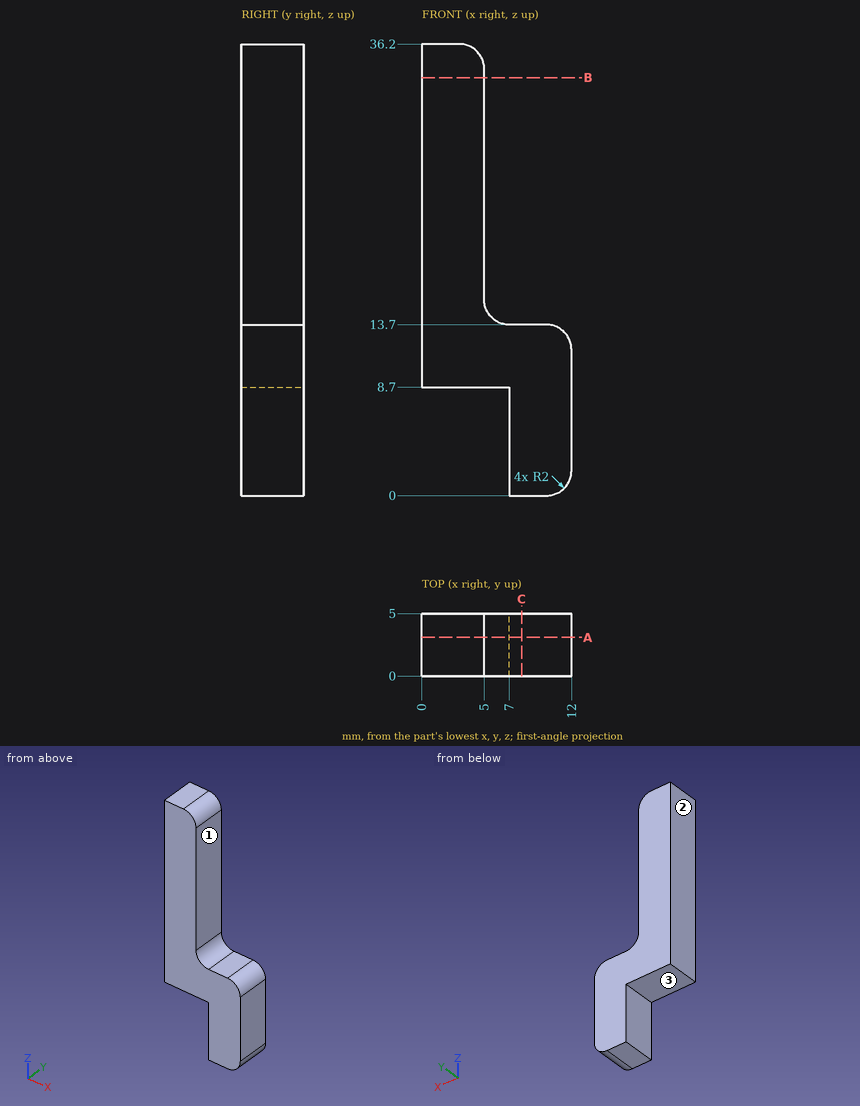
Design review of the part shown in the three views and the two pictorial views. Dimensions are in mm from the part's minimum x, y and z. A direction names the side the tool comes from. Coordinates: 2 decimals unless noted, no trailing zeros. Order: outer loops, then holes, each group sorted by start corner. A loop starts at its lowest first (then second) coordinate and runs counter-clockwise, first axis right, second up. Notation, with made-up numbers: (40.5, -31.5) - (89.5, -31.5) arc R7 cw to (89.5, -25.5) - close; hole circle Ø11 at (41.25, 3.5). An arc over 180 degrees is marked (long way). One line per question, with ' | ' between items.
Q1. Consider section C-C, the plane x = 8. Give the boundary of the cut face in (y, z).
Answer key:
outline: (0, 0) - (5, 0) - (5, 13.7) - (0, 13.7) - close
Q2. For the marked faces 1, 2 and 3, list the 3-axis set-ups (+Z, -Z, +X, -X, +Y, -Y) from which the entire face can be reached by the end or side of a thin tool; tool diameter is ignored.
Answer key:
face 1: +Z, +X, +Y, -Y | face 2: +Z, -Z, -X, +Y, -Y | face 3: -Z, -X, +Y, -Y
Q3. Clearance check with flat-ended pins moving along their axes: pin 1 Ø2.5 at (y, z) = (2, 2.5) entering from -X; pin 2 Ø2.5 at (y, z) = (1.5, 25.5) entering from +X; pin 3 Ø1 at (x, y) = (6.5, 1.5) entering from +Z. State where each tip first meets the part, or that it passes through.
Answer key:
pin 1: stops at x = 7 | pin 2: stops at x = 5 | pin 3: stops at z = 13.97
Q4. To check wall thickness, follow line 1 along X through (y, z) = (0.55, 26); line 2 along Z through (x, y) = (1.25, 0.5); line 3 along X through (y, z) = (3.5, 7). State the ranges of each line that lie inside material, in increasing order.
Answer key:
line 1: x = 0 to 5 | line 2: z = 8.7 to 36.2 | line 3: x = 7 to 12
Q5. Consider section B-B, the plane z = 33.5. Give the boundary of the cut face in (x, y).
Answer key:
outline: (0, 0) - (5, 0) - (5, 5) - (0, 5) - close
Q6. Consider section A-A, the plane y = 3.1. Give the boundary of the cut face in (x, z), then the cut area to 3 significant figures.
Answer key:
outline: (0, 8.7) - (7, 8.7) - (7, 0) - (10, 0) arc R2 ccw to (12, 2) - (12, 11.7) arc R2 ccw to (10, 13.7) - (7, 13.7) arc R2 cw to (5, 15.7) - (5, 34.2) arc R2 ccw to (3, 36.2) - (0, 36.2) - close | area: 214 mm2
